Check sheet for the modelled part. Datum: model origin and axes. Units: mm. Face numbers are marked on the shaded views. A direction names the side the tool comes from. Coordinates: 2 decimals unless noted, no trailing zeros. Write each loop counter-clockwise with the first axis right and the second up, starting at its lowest first coordinate (ties: lowest second). Pieces come first, ordered by that corner, then holes. Notation, with made-up numbers: (70.5, 1.25) -> (109.5, 1.25) arc R21 cw to (109.5, 38.25) -> close; hole circle Ø1 at (89, 46.5). An arc over 180 degrees is marked (long way). Put each result on its own line as item: value.
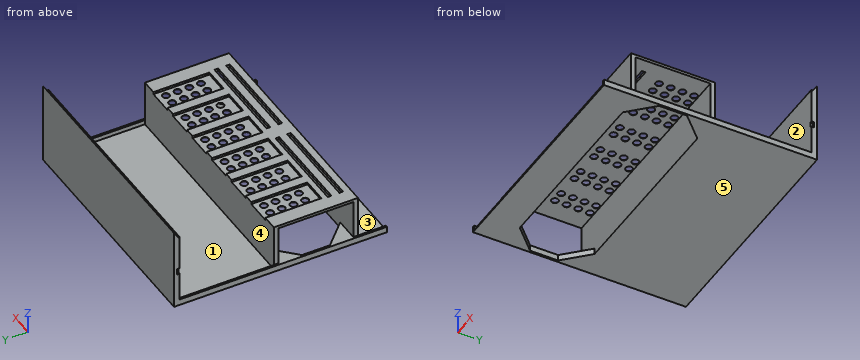
```python
from build123d import *

# Parameters (mm, degrees)
BOSS_EXTRUDE1_DEPTH = 2.6
SKETCH2_W           = 100.4
SKETCH2_H           = 2.4
BOSS_EXTRUDE2_DEPTH = 30
LPATTERN1_COUNT     = 2
LPATTERN1_PITCH     = 15
SKETCH5_W           = 2.6
SKETCH5_H           = 2
BOSS_EXTRUDE4_DEPTH = 98.8
SKETCH7_W           = 0.8
SKETCH7_H           = 2.6
CUT_EXTRUDE1_DEPTH  = 90
SKETCH8_W           = 0.8
SKETCH8_H           = 2.6
CUT_EXTRUDE2_DEPTH  = 90
BOSS_EXTRUDE5_DEPTH = 100.4
SKETCH11_W          = 10.8
SKETCH11_H          = 24
CUT_EXTRUDE3_DEPTH  = 1
LPATTERN2_COUNT     = 6
LPATTERN2_PITCH     = 15
SKETCH13_W          = 98.8
SKETCH13_H          = 32
CUT_EXTRUDE4_DEPTH  = 10
CHAMFER1_SIZE       = 10
SKETCH15_R          = 1.5
CUT_EXTRUDE17_DEPTH = 10
SKETCH18_W          = 40
SKETCH18_H          = 1.6
CUT_EXTRUDE18_DEPTH = 10


with BuildPart() as part:
    # Sketch1 → Boss-Extrude1 (new body)
    with BuildSketch(Plane.XY):
        Polygon((-13.007233288, 0), (-13.007233288, 90), (85.792766712, 90), (85.792766712, 0), (86.592766712, 0), (86.592766712, 91.2), (-13.807233288, 91.2), (-13.807233288, 0), align=None)
    boss_extrude1 = extrude(amount=BOSS_EXTRUDE1_DEPTH)

    # Sketch2 → Boss-Extrude2 (add)
    with BuildSketch(Plane.XY.offset(2.6)):
        with Locations((36.392766712, 90)):
            Rectangle(SKETCH2_W, SKETCH2_H)
    extrude(amount=BOSS_EXTRUDE2_DEPTH)

    # LPattern1: Boss-Extrude1 ×2
    with Locations(*[(0, 0, i * LPATTERN1_PITCH) for i in range(1, LPATTERN1_COUNT)]):
        add(boss_extrude1)

    # Sketch5 → Boss-Extrude4 (add)
    with BuildSketch(Plane.ZY.offset(-85.792766712)):
        Polygon((20.6, 12), (20.6, 48), (17.6, 48), (17.6, 46), (19.4, 46), (19.4, 14), (17.6, 14), (17.6, 12), align=None)
        Polygon((15, 46), (15, 48), (5.6, 48), (0.6, 48), (0.6, 90), (0, 90), (0, 48.076108626), (0, 12.076108626), (0, 0), (0.6, 0), (0.6, 12), (5.6, 12), (15, 12), (15, 14), (0.6, 14), (0.6, 46), align=None)
        with Locations((16.3, 13)):
            Rectangle(SKETCH5_W, SKETCH5_H)
        with Locations((16.3, 47)):
            Rectangle(SKETCH5_W, SKETCH5_H)
    extrude(amount=BOSS_EXTRUDE4_DEPTH)

    # Sketch7 → Cut-Extrude1 (cut)
    with BuildSketch(Plane.XZ):
        with Locations((-13.407233288, 16.3)):
            Rectangle(SKETCH7_W, SKETCH7_H)
    extrude(amount=-CUT_EXTRUDE1_DEPTH, mode=Mode.SUBTRACT)

    # Sketch8 → Cut-Extrude2 (cut)
    with BuildSketch(Plane.XZ):
        with Locations((86.192766712, 16.3)):
            Rectangle(SKETCH8_W, SKETCH8_H)
    extrude(amount=-CUT_EXTRUDE2_DEPTH, mode=Mode.SUBTRACT)

    # Sketch10 → Boss-Extrude5 (add)
    with BuildSketch(Plane(origin=(86.592766712, 0, 0), x_dir=(0, 0, -1), z_dir=(1, 0, 0))):
        Polygon((-35.4, 91.2), (-32.6, 89.4), (-32.6, 91.2), align=None)
    extrude(amount=-BOSS_EXTRUDE5_DEPTH)

    # Sketch11 → Cut-Extrude3 (cut)
    with BuildSketch(Plane.XY.offset(20.6)):
        with Locations((-1.107233288, 36)):
            Rectangle(SKETCH11_W, SKETCH11_H)
    cut_extrude3 = extrude(amount=-CUT_EXTRUDE3_DEPTH, mode=Mode.SUBTRACT)

    # LPattern2: Cut-Extrude3 ×6
    with Locations(*[(i * LPATTERN2_PITCH, 0, 0) for i in range(1, LPATTERN2_COUNT)]):
        add(cut_extrude3, mode=Mode.SUBTRACT)

    # Sketch13 → Cut-Extrude4 (cut)
    with BuildSketch(Plane.XY.offset(0.6)):
        with Locations((36.392766712, 30)):
            Rectangle(SKETCH13_W, SKETCH13_H)
    extrude(amount=-CUT_EXTRUDE4_DEPTH, mode=Mode.SUBTRACT)

    # Chamfer1
    chamfer1_edges = [part.edges().sort_by_distance(p)[0] for p in [
        (85.792766712, 46, 1.3),
        (-13.007233288, 14, 1.3),
        (-13.007233288, 46, 1.3),
        (85.792766712, 14, 1.3),
    ]]
    chamfer(chamfer1_edges, length=CHAMFER1_SIZE)

    # Sketch15 → Cut-Extrude17 (cut)
    with BuildSketch(Plane.XY.offset(19.6)):
        with Locations((-3.507233288, 44.31513876)):
            Circle(SKETCH15_R)
        with Locations((1.292766712, 44.31513876)):
            Circle(SKETCH15_R)
        with Locations((11.492766712, 44.31513876)):
            Circle(SKETCH15_R)
        with Locations((16.292766712, 44.31513876)):
            Circle(SKETCH15_R)
        with Locations((26.492766712, 44.31513876)):
            Circle(SKETCH15_R)
        with Locations((31.292766712, 44.31513876)):
            Circle(SKETCH15_R)
        with Locations((41.492766712, 44.31513876)):
            Circle(SKETCH15_R)
        with Locations((46.292766712, 44.31513876)):
            Circle(SKETCH15_R)
        with Locations((56.492766712, 44.31513876)):
            Circle(SKETCH15_R)
        with Locations((61.292766712, 44.31513876)):
            Circle(SKETCH15_R)
        with Locations((71.492766712, 44.31513876)):
            Circle(SKETCH15_R)
        with Locations((76.292766712, 44.31513876)):
            Circle(SKETCH15_R)
        with Locations((11.492766712, 39.31513876)):
            Circle(SKETCH15_R)
        with Locations((16.292766712, 39.31513876)):
            Circle(SKETCH15_R)
        with Locations((26.492766712, 39.31513876)):
            Circle(SKETCH15_R)
        with Locations((31.292766712, 39.31513876)):
            Circle(SKETCH15_R)
        with Locations((41.492766712, 39.31513876)):
            Circle(SKETCH15_R)
        with Locations((46.292766712, 39.31513876)):
            Circle(SKETCH15_R)
        with Locations((56.492766712, 39.31513876)):
            Circle(SKETCH15_R)
        with Locations((61.292766712, 39.31513876)):
            Circle(SKETCH15_R)
        with Locations((71.492766712, 39.31513876)):
            Circle(SKETCH15_R)
        with Locations((76.292766712, 39.31513876)):
            Circle(SKETCH15_R)
        with Locations((11.492766712, 34.31513876)):
            Circle(SKETCH15_R)
        with Locations((16.292766712, 34.31513876)):
            Circle(SKETCH15_R)
        with Locations((26.492766712, 34.31513876)):
            Circle(SKETCH15_R)
        with Locations((31.292766712, 34.31513876)):
            Circle(SKETCH15_R)
        with Locations((41.492766712, 34.31513876)):
            Circle(SKETCH15_R)
        with Locations((46.292766712, 34.31513876)):
            Circle(SKETCH15_R)
        with Locations((56.492766712, 34.31513876)):
            Circle(SKETCH15_R)
        with Locations((61.292766712, 34.31513876)):
            Circle(SKETCH15_R)
        with Locations((71.492766712, 34.31513876)):
            Circle(SKETCH15_R)
        with Locations((76.292766712, 34.31513876)):
            Circle(SKETCH15_R)
        with Locations((11.492766712, 29.31513876)):
            Circle(SKETCH15_R)
        with Locations((16.292766712, 29.31513876)):
            Circle(SKETCH15_R)
        with Locations((26.492766712, 29.31513876)):
            Circle(SKETCH15_R)
        with Locations((31.292766712, 29.31513876)):
            Circle(SKETCH15_R)
        with Locations((41.492766712, 29.31513876)):
            Circle(SKETCH15_R)
        with Locations((46.292766712, 29.31513876)):
            Circle(SKETCH15_R)
        with Locations((56.492766712, 29.31513876)):
            Circle(SKETCH15_R)
        with Locations((61.292766712, 29.31513876)):
            Circle(SKETCH15_R)
        with Locations((71.492766712, 29.31513876)):
            Circle(SKETCH15_R)
        with Locations((76.292766712, 29.31513876)):
            Circle(SKETCH15_R)
        with Locations((-3.507233288, 39.31513876)):
            Circle(SKETCH15_R)
        with Locations((1.292766712, 39.31513876)):
            Circle(SKETCH15_R)
        with Locations((-3.507233288, 34.31513876)):
            Circle(SKETCH15_R)
        with Locations((1.292766712, 34.31513876)):
            Circle(SKETCH15_R)
        with Locations((-3.507233288, 29.31513876)):
            Circle(SKETCH15_R)
        with Locations((1.292766712, 29.31513876)):
            Circle(SKETCH15_R)
    extrude(amount=-CUT_EXTRUDE17_DEPTH, mode=Mode.SUBTRACT)

    # Sketch18 → Cut-Extrude18 (cut)
    with BuildSketch(Plane.XY.offset(20.6)):
        with Locations((59.792766712, 20.8)):
            Rectangle(SKETCH18_W, SKETCH18_H)
        with Locations((12.992766712, 20.8)):
            Rectangle(SKETCH18_W, SKETCH18_H)
        with Locations((59.792766712, 15.8)):
            Rectangle(SKETCH18_W, SKETCH18_H)
        with Locations((12.992766712, 15.8)):
            Rectangle(SKETCH18_W, SKETCH18_H)
    extrude(amount=-CUT_EXTRUDE18_DEPTH, mode=Mode.SUBTRACT)


solid = part.part
```
Q1. Cross-section at D-D (x = 36). Record the cut outline in (y, z), plus the area to 3 significant figures.
Recorded:
outline: (0, 0) -> (14, 0) -> (14, 19.4) -> (46, 19.4) -> (46, 0) -> (91.2, 0) -> (91.2, 35.4) -> (89.4, 32.6) -> (88.8, 32.6) -> (88.8, 2.6) -> (90, 2.6) -> (90, 0.6) -> (48, 0.6) -> (48, 20.6) -> (12, 20.6) -> (12, 0.6) -> (0, 0.6) -> close
area: 231 mm2
Q2. Tool access check on the marked faces 3, 4 and 5. Record the directions out of +Z, -Z, +X, -X, +Y, -Y that give a thin tool (end or side, any length) a straight path to the whole face; none if there is none.
Recorded:
face 3: +Z, -Y
face 4: +Z
face 5: -Z, +X, -X, +Y, -Y
Q3. Mould release check, pull along X, two halves, no side actions. Record for the marked faces 1 and 2: released by +X, released by -X, zero draft, split by the parting line, or undercut.
Recorded:
face 1: undercut
face 2: zero draft
Q4. Material ranges on line 1 along Y through (x, z) = (20, 6); line 2 along Y through (x, z) = (78, 2); line 3 along Y through (x, z) = (54, 29.5), recorded low to high.
Recorded:
line 1: y = 12 to 14, 46 to 48, 88.8 to 91.2
line 2: y = 12 to 16.21, 43.79 to 48, 90 to 91.2
line 3: y = 88.8 to 91.2
Q5. Cross-section at B-B (x = 6). Record the cut outline in (y, z).
Recorded:
outline: (0, 0) -> (14, 0) -> (14, 19.4) -> (15, 19.4) -> (15, 20.6) -> (12, 20.6) -> (12, 0.6) -> (0, 0.6) -> close; (16.6, 19.4) -> (20, 19.4) -> (20, 20.6) -> (16.6, 20.6) -> close; (21.6, 19.4) -> (46, 19.4) -> (46, 0) -> (91.2, 0) -> (91.2, 35.4) -> (89.4, 32.6) -> (88.8, 32.6) -> (88.8, 2.6) -> (90, 2.6) -> (90, 0.6) -> (48, 0.6) -> (48, 20.6) -> (21.6, 20.6) -> close
Q6. Cross-section at C-C (y = 61). Record the cut outline in (x, z), plus the area to 3 significant figures.
Recorded:
outline: (-13.81, 0) -> (86.59, 0) -> (86.59, 2.6) -> (85.79, 2.6) -> (85.79, 0.6) -> (-13.01, 0.6) -> (-13.01, 2.6) -> (-13.81, 2.6) -> close
area: 63.4 mm2
Q7. Depth check by flat-ended pin: P1, Ø10, axis at x = 57.5, z = 13, coming from the -Y side; P2, Ø4, axis at x = 76.29, y = 29.32, coming from the -Z side; P3, Ø3, axis at x = 52.5, y = 75.5, coming from the +Z side. Enter the tip coordinate at first touch or a pass-through.
Recorded:
P1: stops at y = 12
P2: stops at z = 19.4
P3: stops at z = 0.6
Q8. Cross-section at A-A (z = 9.5). Record the cut outline in (x, y).
Recorded:
outline: (-13.81, 88.8) -> (86.59, 88.8) -> (86.59, 91.2) -> (-13.81, 91.2) -> close; (-13.01, 12) -> (85.79, 12) -> (85.79, 14) -> (-13.01, 14) -> close; (-13.01, 46) -> (85.79, 46) -> (85.79, 48) -> (-13.01, 48) -> close
